```python
from build123d import *

# Parameters (mm, degrees)
SKETCH3_R          = 1.5
SKETCH3_R_2        = 3.25
SKETCH3_R_3        = 2
SKETCH3_R_4        = 1.25
CUT_EXTRUDE1_DEPTH = 10


with BuildPart() as part:
    # Sketch1 → Revolve1 (revolve)
    with BuildSketch(Plane.XY, mode=Mode.PRIVATE) as revolve1_sk:
        Polygon((11.05, 0), (11.05, 8), (13.05, 8), (13.05, 3.969255392), (22, 3.969255392), (22, 0), align=None)
    revolve(revolve1_sk.sketch.rotate(Axis((0, 0, 0), (0, 1, 0)), 90), axis=Axis((0, 0, 0), (0, 1, 0)))

    # Sketch3 → Cut-Extrude1 (cut)
    with BuildSketch(Plane(origin=(0, 0, 0), x_dir=(1, 0, 0), z_dir=(0, 1, 0))):
        with Locations(Location((16.5, 0, 0), (0, 0, 270))):
            Circle(SKETCH3_R)
        with Locations(Location((-8.25, -14.289419162, 0), (0, 0, 270))):
            Circle(SKETCH3_R)
        with Locations(Location((-8.25, 14.289419162, 0), (0, 0, 270))):
            Circle(SKETCH3_R)
        with Locations(Location((11.66726189, -11.66726189, 0), (0, 0, 270))):
            Circle(SKETCH3_R_2)
        with Locations(Location((14.289419162, 8.25, 0), (0, 0, 270))):
            Circle(SKETCH3_R_3)
        with Locations(Location((0, 16.5, 0), (0, 0, 270))):
            Circle(SKETCH3_R_3)
        with Locations(Location((0, -16.5, 0), (0, 0, 270))):
            Circle(SKETCH3_R_4)
        with BuildLine():
            Line((-14, -7), (-14, 7))
            ThreePointArc((-14, 7), (-16.5, 9.5), (-19, 7))
            Line((-19, 7), (-19, -7))
            ThreePointArc((-19, -7), (-16.5, -9.5), (-14, -7))
        make_face()
    extrude(amount=CUT_EXTRUDE1_DEPTH, mode=Mode.SUBTRACT)


solid = part.part
```
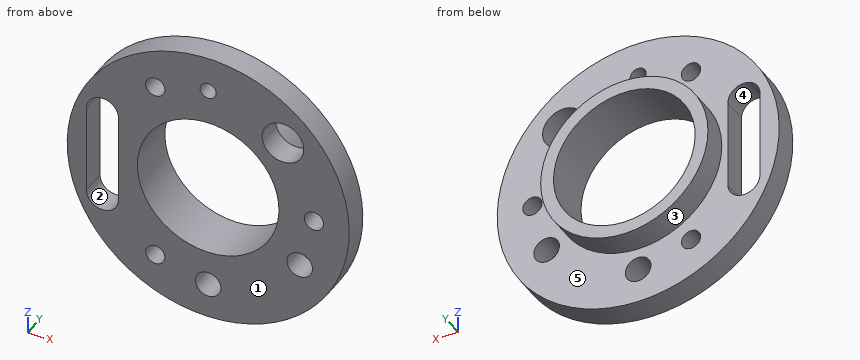
Can you work these out from the model? Positions are in its coordinate system, mm. Face numbers are marked on the shaded views. A direction names the side the tool comes from. Coordinates: 2 decimals unless noted, no trailing zeros. Loops run counter-clockwise (first coordinate to the right, second up) from the corner with the lowest first, then second, coordinate; pieces in that order, holes last.
1) For pin 1 (4 mm diameter, centred on x = 16.5, z = 0, fed in from +Y); pin 2 (2 mm diameter, centred on y = 2.5, z = 3, fed in from +X); pin 3 (2 mm diameter, centred on y = 1.5, z = -1, fed in from -X), each with a flat end and sliding along its axis, tell me the tip position at first contact or that it passes through.
2) Imagine slicing it at B-B on x = -16.5. List the corners of the cut face in (y, z) for me, plus the area to 3 significant figures.
3) Imagine slicing it at D-D on z = -8.25. List the corners of the cut face in (x, y) for me, plus the area to 3 significant figures.
4) Imagine slicing it at A-A on x = 0. List the corners of the cut face in (y, z) for me, plus the area to 3 significant figures.
5) Which directions (+Z, -Z, +X, -X, +Y, -Y) give clear straight access to the entire face, cutting with the end or side of a thin tool? Please do the marked faces 1 and 2.
6) Imagine slicing it at C-C on z = -3.5. List the corners of the cut face in (x, y) for me.
7) Thinking about a two-plate mould opening in X: for the marked faces 3, 4 and 5, which applies, pulls with the +X half, pulls with the -X half, needs draft (parallel to the pull), parting line crosses it, or undercut?
8) I need wall thicknesses on probe 1 along X at (y, z) = (1.5, 0); probe 2 along Z at (x, y) = (-8.25, 1.4); probe 3 along X at (y, z) = (3.25, -7). Which ranges of each line are inside material? Lowest first, please.
Completed:
1. pin 1: stops at y = 3.97
1. pin 2: stops at x = 21.91
1. pin 3: stops at x = -22
2. outline: (0, -14.55) - (3.97, -14.55) - (3.97, -9.5) - (0, -9.5) - close; (0, 9.5) - (3.97, 9.5) - (3.97, 14.55) - (0, 14.55) - close
2. area: 40.1 mm2
3. outline: (-20.39, 0) - (-18.67, 0) - (-18.67, 3.97) - (-20.39, 3.97) - close; (-14.33, 0) - (-7.35, 0) - (-7.35, 8) - (-10.11, 8) - (-10.11, 3.97) - (-14.33, 3.97) - close; (7.35, 0) - (12.29, 0) - (12.29, 3.97) - (10.11, 3.97) - (10.11, 8) - (7.35, 8) - close; (16.29, 0) - (20.39, 0) - (20.39, 3.97) - (16.29, 3.97) - close
3. area: 92.7 mm2
4. outline: (0, -22) - (3.97, -22) - (3.97, -18.5) - (0, -18.5) - close; (0, -14.5) - (3.97, -14.5) - (3.97, -13.05) - (8, -13.05) - (8, -11.05) - (0, -11.05) - close; (0, 11.05) - (8, 11.05) - (8, 13.05) - (3.97, 13.05) - (3.97, 15.25) - (0, 15.25) - close; (0, 17.75) - (3.97, 17.75) - (3.97, 22) - (0, 22) - close
4. area: 77.2 mm2
5. face 1: +Z, -Z, +X, -X, -Y
5. face 2: +Y, -Y
6. outline: (-21.72, 0) - (-19, 0) - (-19, 3.97) - (-21.72, 3.97) - close; (-14, 0) - (-10.48, 0) - (-10.48, 8) - (-12.57, 8) - (-12.57, 3.97) - (-14, 3.97) - close; (10.48, 0) - (21.72, 0) - (21.72, 3.97) - (12.57, 3.97) - (12.57, 8) - (10.48, 8) - close
7. face 3: parting line crosses it
7. face 4: undercut
7. face 5: needs draft
8. probe 1: x = -22 to -19, -14 to -11.05, 11.05 to 15, 18 to 22
8. probe 2: z = -20.39 to -15.79, -12.79 to -7.35, 7.35 to 12.79, 15.79 to 20.39
8. probe 3: x = -20.86 to -19, -14 to -8.55, 8.55 to 12.73, 15.85 to 20.86
